The drawing under review shows one solid part. Ordinate dimensions are in mm from its lowest x, y, z. A direction names the side the tool comes from. Coordinates: 2 decimals unless noted, no trailing zeros. Order: outer loops, then holes, each group sorted by start corner. A loop starts at its lowest first (then second) coordinate and runs counter-clockwise, first axis right, second up.
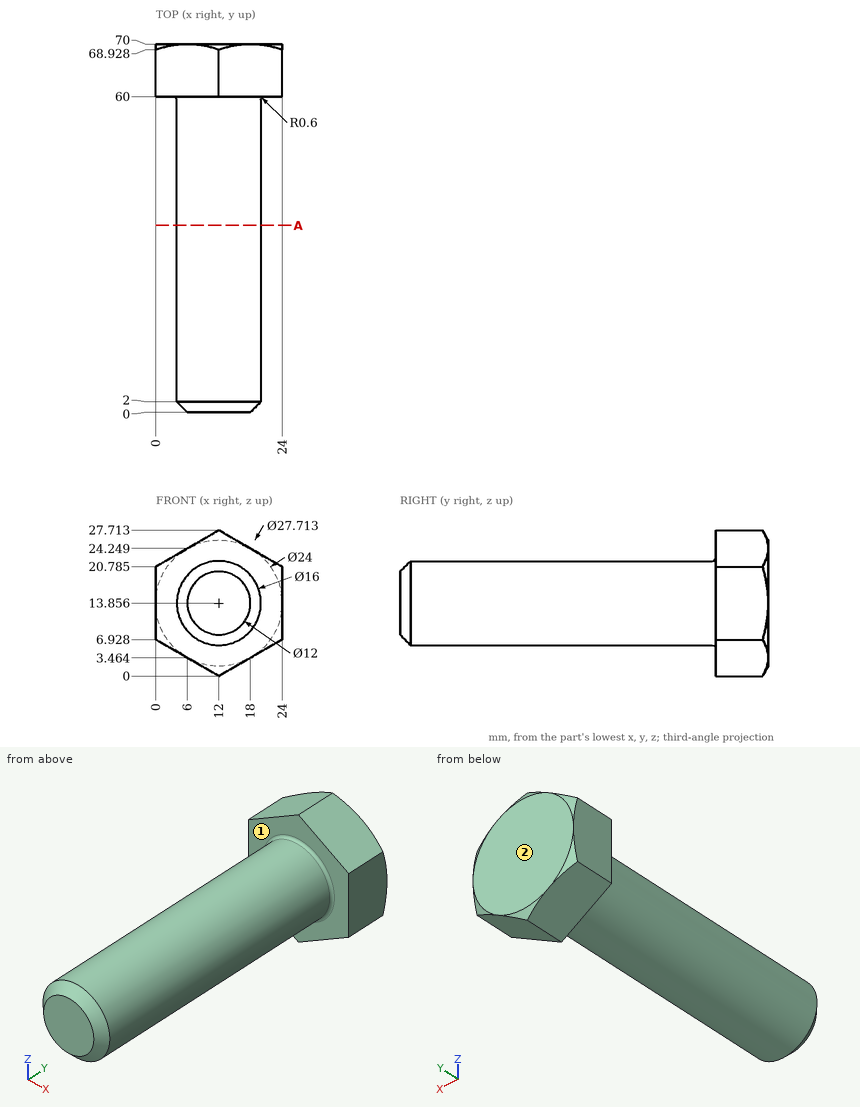
(1) Tool access review of the marked faces 1 and 2: name each direction out of +Z, -Z, +X, -X, +Y, -Y from which nothing blocks a thin tool from reaching the whole face with its end or side.
(2) Insertion check: pin 1 Ø3 at (x, y) = (15.5, 46.5) entering from +Z; pin 2 Ø10 at (y, z) = (17.5, 6.5) entering from +X (1 decimal); pin 3 Ø5 at (y, z) = (8.5, 9.5) entering from -X; pin 4 Ø3 at (y, z) = (52, 4) entering from -X. Each pin has a flat end and moves straight along its axis. Give the tip position at first contact, or say it passes through.
(3) Consider section A-A (y = 35.5). Give the boundary of the cut face in (x, z), then the cut area to 3 significant figures.
(4) Wall thickness on line 1 (Y direction, x = 19.5, z = 22.25); line 2 (X direction, y = 39, z = 14.25); line 3 (Z direction, x = 6.5, y = 22) (1 decimal): over which ranges is each line inside the solid? List them lowest first.
Findings:
1. face 1: -Y
1. face 2: +Z, -Z, +X, -X, +Y
2. pin 1: stops at z = 21.6
2. pin 2: stops at x = 19.6
2. pin 3: stops at x = 4.22
2. pin 4: passes through
3. outline: circle Ø16 at (12, 13.86)
3. area: 201 mm2
4. line 1: y = 60 to 70
4. line 2: x = 4.01 to 19.99
4. line 3: z = 8 to 19.7
